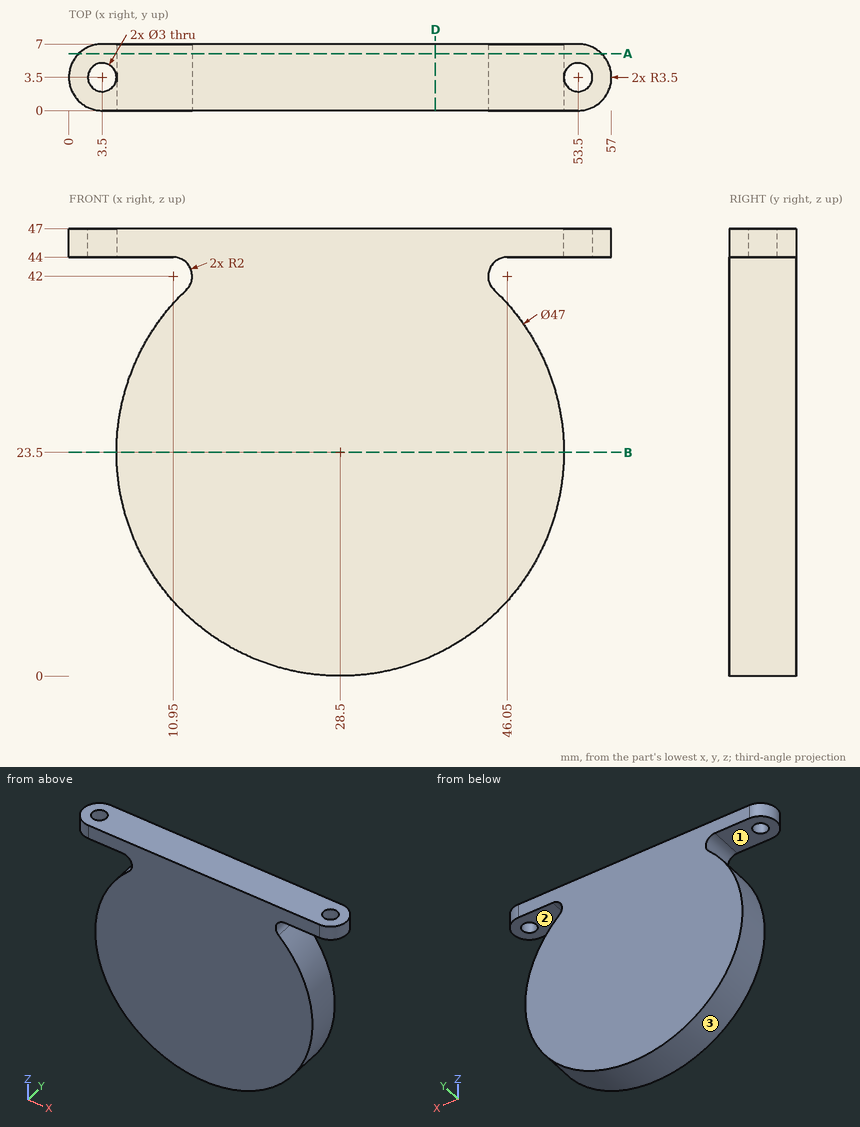
For this review, use the dimensioned drawing (mm, ordinates from the lowest corner) and the shaded views. A direction names the side the tool comes from. Round coordinates to 2 decimals unless told otherwise and drop trailing zeros. Order: outer loops, then holes, each group sorted by start corner. A loop starts at its lowest first (then second) coordinate and runs counter-clockwise, first axis right, second up. Notation, with made-up numbers: M 84.25,59.25 L 142.25,59.25 A29 ccw 142.25,83.25 Z; hole C 71,60 d4. An arc over 180 degrees is marked long. Write each question's results on one line, items separated by ' | '. Start each with the question number.
1. Add section A-A (y = 6). State the section outline as (x, z) points, then the cut area to 3 significant figures.
2. Add section B-B (z = 23.5). State the section outline as (x, y) points, then the cut area to 3 significant figures.
3. Tool access review of the marked faces 1, 2 and 3: name each direction out of +Z, -Z, +X, -X, +Y, -Y from which nothing blocks a thin tool from reaching the whole face with its end or side.
4. Clearance check with flat-ended pins moving along their axes: pin 1 Ø1.5 at (y, z) = (3.5, 29) entering from -X (3 decimals); pin 2 Ø3.5 at (x, y) = (7.5, 4) entering from -Z; pin 3 Ø2 at (x, z) = (19, 17.5) entering from -Y; pin 4 Ø2 at (x, y) = (49, 3.5) entering from -Z (1 decimal). State where each tip first meets the part, or that it passes through.
5. Add section D-D (x = 38.5). State the section outline as (y, z) points.
6. To check wall thickness, follow L1, parallel to Y at x = 53.5, z = 46.1; L2, parallel to Z at x = 14, y = 4; L3, parallel to Z at x = 7.5, y = 0.5. State the ranges of each line that lie inside material, in increasing order. Write a range as [from, to].
Output values:
1) outline: M 1.05,44 L 10.95,44 A2 cw 12.33,40.55 A23.5 ccw long 44.67,40.55 A2 cw 46.05,44 L 55.95,44 L 55.95,47 L 1.05,47 Z | area: 1,870 mm^2
2) outline: M 5,0 L 52,0 L 52,7 L 5,7 Z | area: 329 mm^2
3) face 1: -X, +Y, -Y | face 2: +X, +Y, -Y | face 3: +Y, -Y
4) pin 1: x = 5.485 | pin 2: z = 10.02 | pin 3: y = 0 | pin 4: z = 10.4
5) outline: M 0,2.23 L 7,2.23 L 7,47 L 0,47 Z
6) L1: [0, 2], [5, 7] | L2: [5.01, 47] | L3: [12.95, 34.05], [44, 47]
